Could you check a few things on this model? Use its own coordinates, in mm. Face numbers are marked on the shaded views. A direction names the side the tool comes from. Round coordinates to 2 decimals unless told otherwise and drop trailing zeros. Loops run counter-clockwise (first coordinate to the right, second up) from the corner with the lowest first, then second, coordinate; pieces in that order, holes last. Notation, with made-up numbers: M 80,55 L 112,55 A13 cw 112,64 Z; hole C -34,-35.5 d1. An arc over 180 degrees is marked long. One line per item, written item: value. Start each with the question number.
Q1. I'm going to push flat-ended pins straight in: pin 1 Ø1.8 at (x, y) = (1, 6) entering from +Z; pin 2 Ø1.6 at (x, z) = (2, -1) entering from +Y; pin 3 Ø1.7 at (x, z) = (3, 2.5) entering from +Y. Where does each tip first touch, or does it pass through?
Q2. Imagine slicing it at A-A (x = -1.1). Give the number of separate pieces and of enclosed holes in the cut face, then the cut area to 3 significant figures.
Q3. Imagine slicing it at D-D (x = 4.25). Please give me the cut outline in (y, z).
Q4. Thinking about a two-plate mould opening in Y: for the marked faces 1, 2 and 3, which applies, released by +Y, released by -Y, zero draft, split by the parting line, or undercut?
Q5. Which directions (+Z, -Z, +X, -X, +Y, -Y) give clear straight access to the entire face, cutting with the end or side of a thin tool? Please do the marked faces 4, 5, 6, 7 and 8.
Q6. Imagine slicing it at B-B (z = -0.5). Please give me the cut outline in (x, y), then the cut area to 3 significant figures.
Q7. Imagine slicing it at C-C (y = 6.75). Please give me the cut outline in (x, z), then the cut area to 3 significant figures.
Q8. Please list where these lines run through material, in increasing order: line 1 along Y through (x, z) = (1, 2.7); line 2 along Z through (x, y) = (3.75, 6.5); line 3 along Z through (x, y) = (-2.5, 0.7).
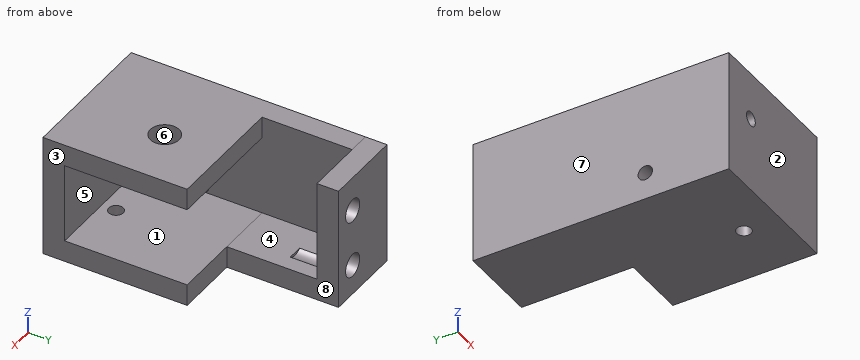
Autodesk Inventor part; units mm, degrees
ref_plane "YZ Plane" through (0, 0, 0) normal (1, 0, 0) x (0, 1, 0)
ref_plane "XZ Plane" through (0, 0, 0) normal (0, 1, 0) x (-1, 0, 0)
ref_plane "XY Plane" through (0, 0, 0) normal (0, 0, 1) x (1, 0, 0)
sketch "Sketch1" plane through (0, 0, 0) normal (0, 1, 0) x (-1, 0, 0)
  line L0 (-5, 5) -> (5, 5)
  line L1 (5, 5) -> (5, -5)
  line L2 (5, -5) -> (-5, -5)
  line L3 (-5, -5) -> (-5, 5)
  line L4 (-5, 5) -> (5, -5) construction
  line L5 (5, 5) -> (-5, -5) construction
  point P0 (0, 0)
  dimension "d0" = 10
  dimension "d1" = 10
extrude "Extrusion1" add sketch "Sketch1" along normal blind 1.5
sketch "Sketch2" plane through (0, 1.5, 0) normal (0, 1, 0) x (1, 0, 0)
  line L0 (-5, -5) -> (-3.5, -5)
  line L1 (-5, -5) -> (5, -5)
  line L2 (-3.5, -5) -> (-3.5, 3.5)
  line L3 (-3.5, 3.5) -> (5, 3.5)
  line L4 (5, 3.5) -> (5, 5)
  line L5 (5, 5) -> (-5, 5)
  line L6 (-5, 5) -> (-5, -5)
  point P0 (0, 0)
  dimension "d4" = 1.5
  dimension "d5" = 8.5
  dimension "d6" = 90
  dimension "d7" = 8.5
  dimension "d8" = 90
  dimension "d9" = 10
  dimension "d10" = 90
extrude "Extrusion2" add sketch "Sketch2" along normal blind 8.5
sketch "Sketch3" plane through (0, 1.5, 0) normal (0, 1, 0) x (1, 0, 0)
  circle A0 centre (-2.5, -0.2) radius 0.5
  line L0 (5, 3.5) -> (-3.5, 3.5)
  line L1 (-3.5, 3.5) -> (-3.5, -5)
  point P0 (0, 0)
  dimension "d13" = 1
  dimension "d14" = 3.7
  dimension "d15" = 1
extrude "Extrusion3" cut sketch "Sketch3" against normal blind 8.5
sketch "Sketch4" plane through (-3.5, 1.5, -3.5) normal (0, 0, 1) x (1, 0, 0)
  circle A0 centre (4.3, 1) radius 0.5
  line L0 (8.5, 0) -> (0, 0)
  line L1 (0, 0) -> (0, 8.5)
  point P0 (3.5, -1.5)
  dimension "d18" = 1
  dimension "d19" = 1
  dimension "d20" = 4.3
extrude "Extrusion4" cut sketch "Sketch4" against normal blind 8.5
sketch "Sketch5" plane through (0, 0, 0) normal (0, -1, 0) x (1, 0, 0)
  circle A0 centre (-2.5, 0.2) radius 0.5
  circle A1 centre (-2.5, 0.2) radius 0.5
  point P0 (0, 0)
  dimension "d23" = 1
  dimension "d24" = 0
extrude "Extrusion5" cut sketch "Sketch5" against normal blind 10
sketch "Sketch6" plane through (-3.5, 1.5, 5) normal (1, 0, 0) x (0, 0, -1)
  circle A0 centre (8.1, 4.3) radius 0.5
  line L0 (0, 0) -> (8.5, 0)
  line L1 (8.5, 0) -> (8.5, 8.5)
  point P0 (5, -1.5)
  dimension "d27" = 1
  dimension "d28" = 4.3
  dimension "d29" = 0.4
extrude "Extrusion6" cut sketch "Sketch6" against normal blind 2
sketch "Sketch7" plane through (-5, 0, 5) normal (0, 0, 1) x (1, 0, 0)
  line L0 (0, 0) -> (10, 0)
  line L1 (10, 0) -> (10, 10)
  line L2 (10, 10) -> (0, 10)
  line L3 (0, 10) -> (0, 0)
  point P0 (5, 0)
extrude "Extrusion7" cut sketch "Sketch7" against normal blind 3
sketch "Sketch8" plane through (-5, 0, 2) normal (0, 0, 1) x (1, 0, 0)
  line L0 (0, 0) -> (10, 0)
  line L1 (10, 0) -> (10, 10)
  line L2 (10, 10) -> (0, 10)
  line L3 (0, 10) -> (0, 0)
  point P0 (5, 0)
extrude "Extrusion8" add sketch "Sketch8" along normal blind 1.5
sketch "Sketch9" plane through (-5, 0, 3.5) normal (0, 0, 1) x (1, 0, 0)
  circle A0 centre (6, 6) radius 1
  line L0 (0, 0) -> (10, 0)
  line L1 (0, 10) -> (0, 0)
  point P0 (5, 0)
  dimension "d36" = 2
  dimension "d37" = 6
  dimension "d38" = 6
extrude "Extrusion9" cut sketch "Sketch9" against normal blind 1.5
sketch "Sketch11" plane through (0, 10, 0) normal (0, 1, 0) x (1, 0, 0)
  line L0 (-5, 5) -> (-5, -3.5)
  line L1 (-5, -3.5) -> (-3.5, -3.5)
  line L2 (5, -3.5) -> (-5, -3.5)
  line L3 (-3.5, 3.5001) -> (-3.5, -3.5)
  line L4 (-5, 5) -> (0.5, 5)
  line L5 (5, 5) -> (-5, 5)
  line L6 (0.5, 5) -> (0.5, 3.5001)
  line L7 (0.5, 3.5001) -> (-3.5, 3.5001)
  point P0 (0, 0)
  dimension "d44" = 1.5
  dimension "d45" = 5.5
extrude "Extrusion10" add sketch "Sketch11" along normal blind 6.25
sketch "Sketch12" plane through (0, 16.25, 0) normal (0, 1, 0) x (1, 0, 0)
  line L0 (0.5, 3.5001) -> (-5, 3.5001)
  line L1 (-5, 3.5001) -> (-5, 5)
  line L2 (-5, 5) -> (0.5, 5)
  line L3 (0.5, 5) -> (0.5, 3.5001)
  point P0 (0, 0)
extrude "Extrusion11" add sketch "Sketch12" along normal blind 1.5
sketch "Sketch13" plane through (-3.5, 10, -3.5001) normal (0, 0, 1) x (1, 0, 0)
  line L0 (4, 0) -> (4, 7.75)
  line L1 (-1.5, 7.75) -> (4, 7.75)
  line L2 (4, 7.75) -> (4, 6.25)
  line L3 (4, 6.25) -> (-1.5, 6.25)
  line L4 (-1.5, 6.25) -> (-1.5, 7.75)
  point P0 (3.5, -10)
  dimension "d50" = 1.5
extrude "Extrusion12" add sketch "Sketch13" along normal blind 7
sketch "Sketch14" plane through (0, 17.75, 0) normal (0, 1, 0) x (1, 0, 0)
  circle A0 centre (-1.1, -1.1) radius 0.8
  line L0 (-5, 5) -> (-5, -3.4999)
  line L1 (0.5, 5) -> (-5, 5)
  point P0 (0, 0)
  dimension "d53" = 1.6
  dimension "d54" = 3.9
  dimension "d55" = 6.1
extrude "Extrusion13" cut sketch "Sketch14" against normal blind 2
sketch "Sketch15" plane through (0, 17.75, 0) normal (0, 1, 0) x (1, 0, 0)
  circle A0 centre (-1.1, 2.9) radius 0.8
  line L0 (-5, 5) -> (-5, -3.4999)
  line L1 (0.5, 5) -> (-5, 5)
  point P0 (0, 0)
  dimension "d58" = 1.6
  dimension "d59" = 3.9
  dimension "d60" = 2.1
extrude "Extrusion14" cut sketch "Sketch15" against normal blind 4
properties part number "Corner2" material "Aluminium 7075"
Report:
1. pin 1: stops at z = -3.5
1. pin 2: stops at y = 1.5
1. pin 3: stops at y = 10
2. separate pieces: 3
2. enclosed holes: 0
2. area: 55.1 mm²
3. outline: M 0,-5 L 10,-5 L 10,-3.5 L 1.5,-3.5 L 1.5,2 L 10,2 L 10,3.5 L 0,3.5 Z
4. face 1: undercut
4. face 2: released by -Y
4. face 3: zero draft
5. face 4: +Z, +X
5. face 5: +X
5. face 6: +Z
5. face 7: +Z, -Z, -X, +Y, -Y
5. face 8: +Z, -Z, +X, +Y
6. outline: M -5,0 L 5,0 L 5,1.5 L -3.5,1.5 L -3.5,16.25 L 0.5,16.25 L 0.5,17.75 L -5,17.75 Z
6. area: 45.4 mm²
7. outline: M -5,-5 L 5,-5 L 5,-3.5 L -3.5,-3.5 L -3.5,2 L 0.34,2 L 0.34,3.5 L -5,3.5 Z; M 1.66,2 L 5,2 L 5,3.5 L 1.66,3.5 Z
7. area: 36.3 mm²
8. line 1: y = 0 to 5, 7 to 10
8. line 2: z = -5 to -3.5, 2 to 3.5
8. line 3: z = -5 to -0.3, 0.7 to 3.5
